```python
from build123d import *

# Parameters (mm, degrees)
SKETCH1_W           = 30
SKETCH1_H           = 60
BOSS_EXTRUDE1_DEPTH = 7.5
SKETCH4_W           = 4
SKETCH4_H           = 60
CUT_EXTRUDE1_DEPTH  = 10
CUT_EXTRUDE2_DEPTH  = 3
SKETCH6_W           = 30
SKETCH6_H           = 15
BOSS_EXTRUDE2_DEPTH = 10
FILLET1_SIZE        = 10
FILLET1_SIZE_2      = 20
BOSS_EXTRUDE3_DEPTH = 25
FILLET2_SIZE        = 20
FILLET2_SIZE_2      = 15
FILLET3_R           = 6
FILLET4_R           = 6


with BuildPart() as part:
    # Sketch1 → Boss-Extrude1 (new, symmetric)
    with BuildSketch(Plane.XY):
        Rectangle(SKETCH1_W, SKETCH1_H)
    extrude(amount=BOSS_EXTRUDE1_DEPTH, both=True)

    # Sketch3 → Cut-Revolve1 (revolve, cut)
    with BuildSketch(Plane(origin=(0, 0, 0), x_dir=(0, 0, -1), z_dir=(1, 0, 0)), mode=Mode.PRIVATE) as cut_revolve1_sk:
        Polygon((-7.5, -5), (-3.5, -5), (-3.5, -3), (3.5, -3), (3.5, -5), (7.5, -5), (7.5, 0), (-7.5, 0), align=None)
    revolve(cut_revolve1_sk.sketch.rotate(Axis((0, 0, 19.169416837), (0, 0, -1)), 270), axis=Axis((0, 0, 19.169416837), (0, 0, -1)), mode=Mode.SUBTRACT)

    # Sketch4 → Cut-Extrude1 (cut)
    with BuildSketch(Plane.ZY.offset(15)):
        with Locations((-0.695939916, 0)):
            Rectangle(SKETCH4_W, SKETCH4_H)
    extrude(amount=-CUT_EXTRUDE1_DEPTH, mode=Mode.SUBTRACT)

    # Sketch5 → Cut-Extrude2 (cut)
    with BuildSketch(Plane.XY.offset(-7.5)):
        Polygon((0, -5.5), (-15, -0.040446486), (-15, 1.364268174), (0, -4.09528534), align=None)
    extrude(amount=CUT_EXTRUDE2_DEPTH, mode=Mode.SUBTRACT)

    # Sketch6 → Boss-Extrude2 (add)
    with BuildSketch(Plane(origin=(0, -30, 0), x_dir=(1, 0, 0), z_dir=(0, 1, 0))):
        Rectangle(SKETCH6_W, SKETCH6_H)
    extrude(amount=-BOSS_EXTRUDE2_DEPTH)

    # Fillet1
    # an asymmetric fillet: 20, 10 mm, written as the material it takes off along each edge
    with BuildSketch(Plane(origin=(-15, -40, 57.5), x_dir=(1, 0, 0), z_dir=(0, 0, -1))) as fillet1_piece_1:
        with BuildLine():
            Bezier((FILLET1_SIZE, 0), (0, 0), (0, -FILLET1_SIZE_2), weights=[1, 0.707106781, 1])
            Line((0, -FILLET1_SIZE_2), (0, 0))
            Line((0, 0), (FILLET1_SIZE, 0))
        make_face()
    extrude(amount=115, mode=Mode.SUBTRACT)

    # Sketch7<5> → Boss-Extrude3 (add)
    with BuildSketch(Plane(origin=(0, 0, -7.5), x_dir=(-1, 0, 0), z_dir=(0, 0, -1))):
        with BuildLine():
            Line((0, -30.068567995), (13.97008046, -28.844444564))
            add(Edge.make_bspline(
                [(5, -40), (6.475610406, -40), (7.888971767, -39.147202629), (9.083741797, -38.42629942), (10.154249723, -37.138694208), (11.86770272, -35.0777557), (13.053604417, -31.855708482), (13.581598782, -30.421169024), (13.97008046, -28.844444564)],
                knots=[0, 0, 0, 0.125, 0.125, 0.25, 0.25, 0.5, 0.5, 0.633954119, 0.633954119, 0.633954119], degree=2))
            Line((5, -40), (0, -40))
            Line((0, -40), (0, -30.068567995))
        make_face()
    extrude(amount=BOSS_EXTRUDE3_DEPTH)

    # Fillet2
    # an asymmetric fillet: 20, 15 mm, written as the material it takes off along each edge
    with BuildSketch(Plane(origin=(15, -40, -57.5), x_dir=(-1, 0, 0), z_dir=(0, 0, 1))) as fillet2_piece_1:
        with BuildLine():
            Bezier((FILLET2_SIZE, 0), (0, 0), (0, -FILLET2_SIZE_2), weights=[1, 0.707106781, 1])
            Line((0, -FILLET2_SIZE_2), (0, 0))
            Line((0, 0), (FILLET2_SIZE, 0))
        make_face()
    extrude(amount=115, mode=Mode.SUBTRACT)

    # Fillet3
    fillet3_edges = [part.edges().sort_by_distance(p)[0] for p in [
        (0, -34.796127772, -7.5),
    ]]
    fillet(fillet3_edges, radius=FILLET3_R)

    # Fillet4
    fillet4_edges = [part.edges().sort_by_distance(p)[0] for p in [
        (-3.984516256, -29.719426147, -7.5),
    ]]
    fillet(fillet4_edges, radius=FILLET4_R)


solid = part.part
```
Part model, mm, in its own coordinate system. A direction names the side the tool comes from. Round coordinates to 2 decimals unless told otherwise and drop trailing zeros. Write each loop counter-clockwise with the first axis right and the second up, starting at its lowest first coordinate (ties: lowest second). Pieces come first, ordered by that corner, then holes. Notation, with made-up numbers: (40.5, -40) -> (77.5, -40) arc R32 ccw to (77.5, -4) -> close; hole circle Ø2 at (-37, -10). An arc over 180 degrees is marked (long way). Return JSON: item names as keys, results as strings. Group by question number.
Q1. Saw through at A-A on y = -7. Write the cut outline in (x, z).
Q2. Probe L1, parallel to Z at x = -8.5, y = -10; L2, parallel to Y at x = 0, z = 6.6; L3, parallel to Z at x = -1.5, y = -13.5. List the from-to ranges inside material, lowest first. Write a range as [from, to].
Q3. Mould opens along X. For faces 1 (the flat face through (-15, 5, -5)), 2 (the flat face through (15, 3, 0)), 3 (the cylindrical face through (-1.08, 4.88, 5.47)) say: pulls with the +X half, pulls with the -X half, needs draft (parallel to the pull), parting line crosses it, or undercut.
Q4. Which spindle directions (+Z, -Z, +X, -X, +Y, -Y) get a long thin tool onto all of the face, cutting with end or side? Do faces 4 (the flat face through (-10, 0, 1.304)), 5 (the flat face through (0.1, 3.3, -3.5)), 6 (the flat face through (-6.887, -29.465, -22.603)), 7 (the flat face through (-0.1, 3.3, 3.5)). Say none if no direction does.
Q5. Pin check, flat tips, straight feed: pin 1 (10.5 mm diameter, centred on y = -33, z = -27.5, fed in from +X); pin 2 (11.5 mm diameter, centred on x = 0, y = 0, fed in from +Z); pin 3 (1.2 mm diameter, centred on x = -7.5, z = -1.5, fed in from +Y); pin 4 (11.5 mm diameter, centred on x = 0, y = 0, fed in from -Z). Stop position of each tip, or through.
Answer:
{
 "1": {"outline": "(-15, -7.5) -> (15, -7.5) -> (15, 7.5) -> (-15, 7.5) -> (-15, 1.3) -> (-5, 1.3) -> (-5, -2.7) -> (-15, -2.7) -> close"},
 "2": {"L1": "[-7.5, -2.7], [1.3, 7.5]", "L2": "[-39.52, -5], [5, 30]", "L3": "[-7.5, 7.5]"},
 "3": {"face 1": "pulls with the -X half", "face 2": "pulls with the +X half", "face 3": "undercut"},
 "4": {"face 4": "-X, +Y", "face 5": "-Z", "face 6": "-Z, +X, +Y", "face 7": "+Z"},
 "5": {"pin 1": "x = 0", "pin 2": "z = 7.5", "pin 3": "y = -30", "pin 4": "z = -7.5"}
}
